from build123d import *

# Parameters (mm, degrees)
SKETCH1_W           = 80
SKETCH1_H           = 60
SKETCH1_W_2         = 50
SKETCH1_H_2         = 16.6
SKETCH1_R           = 1.5875
SKETCH1_W_3         = 65
SKETCH1_H_3         = 18.4
BOSS_EXTRUDE1_DEPTH = 10


with BuildPart() as part:
    # Sketch1 → Boss-Extrude1 (new body)
    with BuildSketch(Plane.XY):
        with Locations((32.5, 17.5)):
            Rectangle(SKETCH1_W, SKETCH1_H)
        with Locations((40, 34.2)):
            Rectangle(SKETCH1_W_2, SKETCH1_H_2, mode=Mode.SUBTRACT)
        with Locations((-3.75, -3.75)):
            Circle(SKETCH1_R, mode=Mode.SUBTRACT)
        with Locations((68.75, -3.75)):
            Circle(SKETCH1_R, mode=Mode.SUBTRACT)
        with Locations((-3.75, 22.15)):
            Circle(SKETCH1_R, mode=Mode.SUBTRACT)
        with Locations((32.5, 9.2)):
            Rectangle(SKETCH1_W_3, SKETCH1_H_3, mode=Mode.SUBTRACT)
        with Locations((68.75, 22.15)):
            Circle(SKETCH1_R, mode=Mode.SUBTRACT)
    extrude(amount=BOSS_EXTRUDE1_DEPTH)


solid = part.part
Here's how the part is built. I have some questions about the finished solid (model axes, mm). A direction names the side the tool comes from. Coordinates: 2 decimals unless noted, no trailing zeros. Order: outer loops, then holes, each group sorted by start corner. A loop starts at its lowest first (then second) coordinate and runs counter-clockwise, first axis right, second up. Notation, with made-up numbers: (-9.75, 20.5) -> (47.25, 20.5) arc R26 ccw to (47.25, 49.5) -> close; hole circle Ø3 at (45, 69). An arc over 180 degrees is marked (long way). Answer in a Markdown table with one row per item.
(1) On a 3-axis mill with a long thin cutter (end or side, diameter ignored), from which of +Z, -Z, +X, -X, +Y, -Y can I reach the whole of each face in a straight line? I mean faces 4 (the face through (40, 42.5, 5)), 5 (the face through (-7.5, 17, 5)). Say none if no direction works.
Answer key:
| item | result |
|---|---|
| face 4 | +Z, -Z |
| face 5 | +Z, -Z, -X, +Y, -Y |
(2) I want a section at A-A on x = 11. List the corners of the cut face in (y, z) for me.
Answer key:
| item | result |
|---|---|
| outline | (-12.5, 0) -> (0, 0) -> (0, 10) -> (-12.5, 10) -> close; (18.4, 0) -> (47.5, 0) -> (47.5, 10) -> (18.4, 10) -> close |
(3) I want a section at D-D on z = 7.25. Count the separate pieces of the cut face and the enclosed holes in it, then the cut area to 3 significant figures.
Answer key:
| item | result |
|---|---|
| separate pieces | 1 |
| enclosed holes | 6 |
| area | 2,740 mm^2 |
(4) I want a section at B-B on y = 29. List the corners of the cut face in (x, z) for me, then the cut area to 3 significant figures.
Answer key:
| item | result |
|---|---|
| outline | (-7.5, 0) -> (15, 0) -> (15, 10) -> (-7.5, 10) -> close; (65, 0) -> (72.5, 0) -> (72.5, 10) -> (65, 10) -> close |
| area | 300 mm^2 |
(5) Thinking about a two-plate mould opening in Y: for faces 1 (the face through (32, 47.5, 5)), 2 (the face through (-5.01, -4.716, 4.93)), 3 (the face through (32, 25, 10)), which applies, +Y half, -Y half, draft (parallel to the pull), parting line (faces both ways), or undercut?
Answer key:
| item | result |
|---|---|
| face 1 | +Y half |
| face 2 | undercut |
| face 3 | draft |
(6) Please list where these lines run through material, in increasing order: probe 1 along Y at (x, z) = (68.75, 5.5); probe 2 along Y at (x, z) = (32, 7); probe 3 along X at (y, z) = (16.5, 5.5).
Answer key:
| item | result |
|---|---|
| probe 1 | -12.5 to -5.34, -2.16 to 20.56, 23.74 to 47.5 |
| probe 2 | -12.5 to 0, 18.4 to 25.9, 42.5 to 47.5 |
| probe 3 | -7.5 to 0, 65 to 72.5 |
(7) I want a section at C-C on x = -3.75. List the corners of the cut face in (y, z) for me.
Answer key:
| item | result |
|---|---|
| outline | (-12.5, 0) -> (-5.34, 0) -> (-5.34, 10) -> (-12.5, 10) -> close; (-2.16, 0) -> (20.56, 0) -> (20.56, 10) -> (-2.16, 10) -> close; (23.74, 0) -> (47.5, 0) -> (47.5, 10) -> (23.74, 10) -> close |
